```python
from build123d import *

# Parameters (mm, degrees)
SKETCH19_R         = 4
CUT_EXTRUDE3_DEPTH = 25.4


with BuildPart() as part:
    # Sketch1 → Revolve1 (revolve)
    with BuildSketch(Plane.XY):
        with BuildLine():
            Line((0, 0), (0, 11.938))
            Line((0, 11.938), (24.765, 11.938))
            ThreePointArc((24.765, 11.938), (26.561051224, 12.681948776), (27.305, 14.478))
            Line((27.305, 14.478), (27.305, 22.933028409))
            Line((27.305, 22.933028409), (28.104406531, 23.876))
            Line((28.104406531, 23.876), (57.15, 23.876))
            Line((57.15, 23.876), (57.15, 49.2125))
            Line((57.15, 49.2125), (759.206, 49.2125))
            Line((759.206, 49.2125), (759.206, 44.1325))
            Line((759.206, 44.1325), (62.23, 44.1325))
            Line((62.23, 44.1325), (62.23, 0))
            Line((62.23, 0), (0, 0))
        make_face()
    revolve(axis=Axis((62.23, 0, 0), (-1, 0, 0)))

    # Sketch16 → Cut-Revolve1 (revolve, cut)
    with BuildSketch(Plane(origin=(0, 0, 0), x_dir=(1, 0, 0), z_dir=(0, 1, 0))):
        Polygon((0, 0), (0, 8.35025), (1.905, 6.556375), (1.905, 0), align=None)
    revolve(axis=Axis((1.905, 0, 0), (-1, 0, 0)), mode=Mode.SUBTRACT)

    # Sketch19 → Cut-Extrude3 (cut)
    with BuildSketch(Plane.ZY.offset(-1.905)):
        Circle(SKETCH19_R)
    extrude(amount=-CUT_EXTRUDE3_DEPTH, mode=Mode.SUBTRACT)

    # Sketch32 → Cut-Revolve6 (revolve, cut)
    with BuildSketch(Plane(origin=(0, 0, 0), x_dir=(1, 0, 0), z_dir=(0, 1, 0)), mode=Mode.PRIVATE) as cut_revolve6_sk:
        Polygon((27.305, 0), (28.575, 0), (27.305, 6.351059428), align=None)
    revolve(cut_revolve6_sk.sketch.rotate(Axis((27.305, 0, 0), (1, 0, 0)), 180), axis=Axis((27.305, 0, 0), (1, 0, 0)), mode=Mode.SUBTRACT)


solid = part.part
```
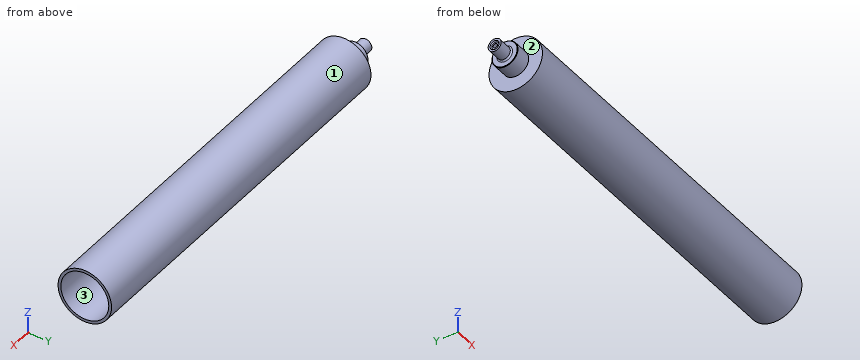
Part model, mm, in its own coordinate system. Face numbers are marked on the shaded views. Round coordinates to 2 decimals unless told otherwise and drop trailing zeros. Loops run counter-clockwise (first coordinate to the right, second up) from the corner with the lowest first, then second, coordinate; pieces in that order, holes last.
Item 1: Mould opens along Z. For the marked faces 1, 2 and 3 say: +Z half, -Z half, draft (parallel to the pull), parting line (faces both ways), or undercut.
Item 2: Cut at B-B, the plane z = -33.5. Give the cut face in (x, y).
Item 3: Drill centre lines: line 1 (Y direction, x = 17, z = 0); line 2 (Z direction, x = 331, y = 0). Where is each one in solid material? Low to high.
Item 4: Drop flat-ended pins along their axis: P1, Ø1.5, axis at x = 414.5, z = 27, coming from the -Y side; P2, Ø1, axis at x = 400.5, y = 29.5, coming from the -Z side; P3, Ø6, axis at x = 658, y = 25.5, coming from the +Z side. Give the stop position or say it passes through.
Item 5: Cut at A-A, the plane x = 584. Give the cut face in (y, z) (1 decimal).
A:
1. face 1: parting line
1. face 2: draft
1. face 3: undercut
2. outline: (57.15, -36.05) - (759.21, -36.05) - (759.21, -28.73) - (62.23, -28.73) - (62.23, 28.73) - (759.21, 28.73) - (759.21, 36.05) - (57.15, 36.05) - close
3. line 1: y = -11.94 to -4, 4 to 11.94
3. line 2: z = -49.21 to -44.13, 44.13 to 49.21
4. P1: stops at y = -41.63
4. P2: stops at z = -39.76
4. P3: stops at z = 43.77
5. outline: circle Ø98.4 at (0, 0); hole circle Ø88.3 at (0, 0)
